```python
from build123d import *

# Parameters (mm, degrees)
F0_W      = 66.3
F0_H      = 24.6
F1_DEPTH  = 2.94
F2_W      = 66.3
F2_H      = 18.75
F3_DEPTH  = 4.5
F5_DEPTH  = 18.75
F7_DEPTH  = 5
F9_DEPTH  = 5
F10_R     = 3.1
F11_DEPTH = 51.751
F12_R     = 5
F13_DEPTH = 21.676
F14_R     = 5
F15_DEPTH = 85.501
F16_R     = 5
F17_R     = 3
F18_R     = 2


with BuildPart() as f1:
    # F0 (on Top) → F1 (new body)
    with BuildSketch(Plane.XY):
        Rectangle(F0_W, F0_H)
    extrude(amount=F1_DEPTH)

    # F2 (on face) → F3 (join)
    with BuildSketch(Plane.XY.offset(2.94)):
        Rectangle(F2_W, F2_H)
    extrude(amount=F3_DEPTH)

    # F4 (on face) → F5 (join, through all)
    with BuildSketch(Plane.XZ.offset(9.375)):
        with BuildLine():
            ThreePointArc((2.75, 94.13226), (0, 23.94), (-2.75, 94.13226))
            Line((-2.75, 94.13226), (-2.75, 123.982605))
            Line((-2.75, 123.982605), (-14, 123.982605))
            Line((-14, 123.982605), (-14, 99.482605))
            ThreePointArc((-14, 99.482605), (-34.828598, 83.879741), (-42.75, 59.09))
            Line((-42.75, 59.09), (-42.75, 7.44))
            Line((-42.75, 7.44), (42.75, 7.44))
            Line((42.75, 7.44), (42.75, 59.09))
            ThreePointArc((42.75, 59.09), (34.828598, 83.879741), (14, 99.482605))
            Line((14, 99.482605), (14, 123.982605))
            Line((14, 123.982605), (2.75, 123.982605))
            Line((2.75, 123.982605), (2.75, 94.13226))
        make_face()
    extrude(amount=-F5_DEPTH)

    # F6 (on face) → F7 (cut)
    with BuildSketch(Plane(origin=(-14, 0, 0), x_dir=(0, -1, 0), z_dir=(-1, 0, 0))):
        Polygon((-3.319764, 105.982605), (3.319764, 105.982605), (6.639528, 111.732605), (3.319764, 117.482605), (-3.319764, 117.482605), (-6.639528, 111.732605), align=None)
    extrude(amount=-F7_DEPTH, mode=Mode.SUBTRACT)

    # F8 (on face) → F9 (cut)
    with BuildSketch(Plane.YZ.offset(14)):
        Polygon((-6.639528, 111.732605), (-3.319764, 105.982605), (3.319764, 105.982605), (6.639528, 111.732605), (3.319764, 117.482605), (-3.319764, 117.482605), align=None)
    extrude(amount=-F9_DEPTH, mode=Mode.SUBTRACT)

    # F10 (on face) → F11 (cut, through all)
    with BuildSketch(Plane(origin=(-9, 0, 0), x_dir=(0, -1, 0), z_dir=(-1, 0, 0))):
        with Locations((0, 111.732605)):
            Circle(F10_R)
    extrude(amount=-F11_DEPTH, mode=Mode.SUBTRACT)

    # F12 (on face) → F13 (cut, through all)
    with BuildSketch(Plane.XZ.offset(9.375)):
        with Locations((0, 9.44)):
            Circle(F12_R)
    extrude(amount=-F13_DEPTH, mode=Mode.SUBTRACT)

    # F14 (on face) → F15 (cut, through all)
    with BuildSketch(Plane(origin=(-42.75, 0, 0), x_dir=(0, -1, 0), z_dir=(-1, 0, 0))):
        with Locations((0, 9.44)):
            Circle(F14_R)
    extrude(amount=-F15_DEPTH, mode=Mode.SUBTRACT)

    # F16
    f16_edges = [f1.edges().sort_by_distance(p)[0] for p in [
        (0, -9.375, 23.94),
    ]]
    fillet(f16_edges, radius=F16_R)

    # F17
    f17_edges = [f1.edges().sort_by_distance(p)[0] for p in [
        (8.375, -9.375, 123.982605),
        (-8.375, -9.375, 123.982605),
        (8.375, 9.375, 123.982605),
        (-8.375, 9.375, 123.982605),
    ]]
    fillet(f17_edges, radius=F17_R)

    # F18
    f18_edges = [f1.edges().sort_by_distance(p)[0] for p in [
        (42.75, -9.375, 33.265),
        (-42.75, -9.375, 33.265),
        (42.75, 9.375, 33.265),
        (-42.75, 9.375, 33.265),
        (14, -9.375, 110.232605),
        (14, 9.375, 110.232605),
        (-14, -9.375, 110.232605),
        (-14, 9.375, 110.232605),
        (-2.75, 2.5, 94.13226),
        (2.75, 2.5, 94.13226),
        (-2.75, 0, 123.982605),
        (2.75, 0, 123.982605),
    ]]
    fillet(f18_edges, radius=F18_R)


solid = f1.part
```
Work out the finished part from the listing and answer in its coordinate system (mm). A direction names the side the tool comes from. Give positions to 0.01 mm unless a question says otherwise; leave off trailing zeros. Loops run counter-clockwise (first coordinate to the right, second up) from the corner with the lowest first, then second, coordinate; pieces in that order, holes last. Notation, with made-up numbers: M 78.5,32 L 82.5,32 A20 cw 82.5,62 Z; hole C -26.75,7.5 d11. An arc over 180 degrees is marked long. One line per item, written item: value. Start each with the question number.
1. Find section A-A (z = 104.5). Give the vertices of the cut face in (x, y) (3 decimals).
2. Which of the six approach directions +Z, -Z, +X, -X, +Y, -Y give full straight-line access (tool end or side, diameter ignored) to faces 1 (the face through (0, -11, 2.94)), 2 (the face through (11.54, 5, 114.57)), 3 (the face through (14, -0.1, 105.6))?
3. Each of these flat-tipped pins is pushed along its axis until it touches: P1, Ø7.5, axis at y = -0.5, z = 110.5, coming from the +X side; P2, Ø3.5, axis at y = 1, z = 4, coming from the +X side; P3, Ø24.5, axis at x = 20, z = 89, coming from the +Y side (3 decimals). Where does it stop, or does it pass through?
4. Determine the mould class of faces 4 (the face through (8.3, 8.5, 123.1)), 5 (the face through (1.48, 2.4, 23.97)), 6 (the face through (-33.15, 0, 3)) for opening direction Z: released by +Z, released by -Z, zero draft, split by the parting line, or undercut.
5. Find section B-B (z = 9.44). Give the vertices of the cut face in (x, y) (3 decimals), and give its area (3 significant figures).
6. Find the intervals of material crossed by probe 1 along Z at (x, y) = (-17, 0); probe 2 along Z at (x, y) = (8.5, 3.5); probe 3 along Z at (x, y) = (12, -4), in increasing order.
7. Find section C-C (x = -18.5). State how many separate pieces and enclosed holes the cut face has, and give its area (3 significant figures).
Reported:
1. outline: M -14,-7.375 A2 ccw -12,-9.375 L -4.75,-9.375 A2 ccw -2.75,-7.375 L -2.75,7.375 A2 ccw -4.75,9.375 L -12,9.375 A2 ccw -14,7.375 Z; M 2.75,-7.375 A2 ccw 4.75,-9.375 L 12,-9.375 A2 ccw 14,-7.375 L 14,7.375 A2 ccw 12,9.375 L 4.75,9.375 A2 ccw 2.75,7.375 Z
2. face 1: +Z, +X, -X, -Y
2. face 2: +X
2. face 3: +Z, +X, +Y, -Y
3. P1: stops at x = 9
3. P2: stops at x = 33.15
3. P3: stops at y = 9.375
4. face 4: released by +Z
4. face 5: undercut
4. face 6: zero draft
5. outline: M -42.75,-7.375 A2 ccw -40.75,-9.375 L -5,-9.375 L -5,-5 L -42.75,-5 Z; M -42.75,5 L -5,5 L -5,9.375 L -40.75,9.375 A2 ccw -42.75,7.375 Z; M 5,-9.375 L 40.75,-9.375 A2 ccw 42.75,-7.375 L 42.75,-5 L 5,-5 Z; M 5,5 L 42.75,5 L 42.75,7.375 A2 ccw 40.75,9.375 L 5,9.375 Z
5. area: 657 mm²
6. probe 1: z = 0 to 4.44, 14.44 to 28.32, 89.86 to 98.31
6. probe 2: z = 0 to 5.87, 13.01 to 24.98, 93.2 to 123.98
6. probe 3: z = 0 to 6.44, 12.44 to 26.05, 92.13 to 107.16, 116.3 to 123.98
7. separate pieces: 2
7. enclosed holes: 1
7. area: 634 mm²
